```python
from build123d import *

# Parameters (mm, degrees)
ESBO_O1_R                  = 25
RESSALTO_EXTRUS_O1_DEPTH   = 30
ESBO_O2_R                  = 35
CORTE_EXTRUS_O1_DEPTH      = 25
ESBO_O3_R                  = 2.9
RESSALTO_EXTRUS_O2_DEPTH   = 6
ESBO_O4_R                  = 3
CORTE_EXTRUS_O2_DEPTH      = 123.727390525
CORTE_EXTRUS_O3_REACH      = 189.931
PADR_OCIRCULAR1_COUNT      = 9
CORTE_EXTRUS_O4_DEPTH      = 123.975657693
CORTE_EXTRUS_O4_DEPTH_BACK = 123.975657693
ESBO_O7_W                  = 10
ESBO_O7_H                  = 6
ESBO_O7_W_2                = 12
ESBO_O7_H_2                = 15
FILETE1_R                  = 1


with BuildPart() as part:
    # Esboço1 → Ressalto-extrusão1 (new body)
    with BuildSketch(Plane(origin=(0, 0, 0), x_dir=(1, 0, 0), z_dir=(0, 1, 0))):
        Polygon((-73.430577701, 42.395163802), (-83.502172006, -14.723685872), (-54.502172006, -64.953159292), (0, -84.790327605), (54.502172006, -64.953159292), (83.502172006, -14.723685872), (73.430577701, 42.395163802), (29, 79.676845164), (-29, 79.676845164), align=None)
        with Locations(Location((0, 0, 0), (0, 0, 270))):
            Circle(ESBO_O1_R, mode=Mode.SUBTRACT)
    extrude(amount=RESSALTO_EXTRUS_O1_DEPTH)

    # Esboço2 → Corte-extrusão1 (cut)
    with BuildSketch(Plane(origin=(0, 30, 0), x_dir=(1, 0, 0), z_dir=(0, 1, 0))):
        Polygon((-79.310129922, -13.984515749), (-51.766010859, -61.692329415), (0, -80.533616515), (51.766010859, -61.692329415), (79.310129922, -13.984515749), (69.74415776, 40.266808257), (27.544119063, 75.676845164), (-27.544119063, 75.676845164), (-69.74415776, 40.266808257), align=None)
        with Locations(Location((0, 0, 0), (0, 0, 270))):
            Circle(ESBO_O2_R, mode=Mode.SUBTRACT)
    extrude(amount=-CORTE_EXTRUS_O1_DEPTH, mode=Mode.SUBTRACT)

    # Esboço3 → Ressalto-extrusão2 (add)
    with BuildSketch(Plane(origin=(0, 30, 0), x_dir=(1, 0, 0), z_dir=(0, 1, 0))):
        with Locations(Location((0, 30, 0), (0, 0, 90))):
            Circle(ESBO_O3_R)
        with Locations(Location((25.980762114, -15, 0), (0, 0, 90))):
            Circle(ESBO_O3_R)
        with Locations(Location((-25.980762114, -15, 0), (0, 0, 90))):
            Circle(ESBO_O3_R)
    extrude(amount=RESSALTO_EXTRUS_O2_DEPTH)

    # Esboço4 → Corte-extrusão2 (cut, through all)
    with BuildSketch(Plane(origin=(0, 30, 0), x_dir=(1, 0, 0), z_dir=(0, 1, 0))):
        with Locations(Location((0, -30, 0), (0, 0, 270))):
            Circle(ESBO_O4_R)
        with Locations(Location((-25.980762114, 15, 0), (0, 0, 270))):
            Circle(ESBO_O4_R)
        with Locations(Location((25.980762114, 15, 0), (0, 0, 270))):
            Circle(ESBO_O4_R)
    extrude(amount=-CORTE_EXTRUS_O2_DEPTH, mode=Mode.SUBTRACT)

    # Esboço5 → Corte-extrusão3 (cut, up to next)
    with BuildSketch(Plane(origin=(0, 0, -79.676845164), x_dir=(-1, 0, 0), z_dir=(0, 0, -1)), mode=Mode.PRIVATE) as corte_extrus_o3_sk1:
        with BuildLine():
            Line((-14.5, 22.5), (14.5, 22.5))
            ThreePointArc((14.5, 22.5), (22, 15), (14.5, 7.5))
            Line((14.5, 7.5), (-14.5, 7.5))
            ThreePointArc((-14.5, 7.5), (-22, 15), (-14.5, 22.5))
        make_face()
    corte_extrus_o3_tool1 = extrude(corte_extrus_o3_sk1.sketch, amount=-CORTE_EXTRUS_O3_REACH, mode=Mode.PRIVATE) & part.part
    corte_extrus_o3 = corte_extrus_o3_tool1.solids().sort_by_distance((0, 15, -79.676845))[0]
    add(corte_extrus_o3, mode=Mode.SUBTRACT)

    # PadrãoCircular1: Corte-extrusão3 ×9 about axis
    padr_ocircular1_axis = Axis((0, 0, 0), (0, 1, 0))
    for i in range(1, PADR_OCIRCULAR1_COUNT):
        add(corte_extrus_o3.rotate(padr_ocircular1_axis, i * 360 / PADR_OCIRCULAR1_COUNT), mode=Mode.SUBTRACT)

    # Esboço7 → Corte-extrusão4 (cut, two sides: drawn at the far end of the back side and taken through both)
    with BuildSketch(Plane(origin=(0, 5, 0), x_dir=(1, 0, 0), z_dir=(0, 1, 0)).offset(-CORTE_EXTRUS_O4_DEPTH_BACK)):
        Polygon((30.672588783, 44.332787011), (38.333033214, 37.904910914), (42.189758872, 42.501177572), (34.529314441, 48.929053669), align=None)
        with Locations((0, 56.676845164)):
            Rectangle(ESBO_O7_W, ESBO_O7_H)
        Polygon((51.993132387, 14.244925111), (53.729614163, 4.396847581), (59.638460681, 5.438736647), (57.901978905, 15.286814177), align=None)
        Polygon((48.985511507, -22.508295563), (43.985511507, -31.168549601), (49.18166393, -34.168549601), (54.18166393, -25.508295563), align=None)
        Polygon((23.05702538, -48.729634591), (13.660099172, -52.149836024), (15.712220032, -57.787991749), (25.10914624, -54.367790316), align=None)
        Polygon((-13.660099172, -52.149836024), (-23.05702538, -48.729634591), (-25.10914624, -54.367790316), (-15.712220032, -57.787991749), align=None)
        Polygon((-43.985511507, -31.168549601), (-48.985511507, -22.508295563), (-54.18166393, -25.508295563), (-49.18166393, -34.168549601), align=None)
        Polygon((-53.729614163, 4.396847581), (-51.993132387, 14.244925111), (-57.901978905, 15.286814177), (-59.638460681, 5.438736647), align=None)
        Polygon((-38.333033214, 37.904910914), (-30.672588783, 44.332787011), (-34.529314441, 48.929053669), (-42.189758872, 42.501177572), align=None)
        Polygon((-23.065208837, -36.822388457), (-32.257742154, -29.10893714), (-41.8995563, -40.599603787), (-32.707022982, -48.313055103), align=None)
        with Locations((0, -50.533616515)):
            Rectangle(ESBO_O7_W_2, ESBO_O7_H_2)
        Polygon((-41.337950118, -13.381555604), (-43.42172825, -1.563862568), (-58.193844545, -4.168585233), (-56.110066413, -15.986278269), align=None)
        Polygon((-40.268205119, 16.320655835), (-34.268205119, 26.71296068), (-47.258586175, 34.21296068), (-53.258586175, 23.820655835), align=None)
        Polygon((-20.356519413, 38.386251025), (-9.080207964, 42.490492745), (-14.210510113, 56.585882056), (-25.486821563, 52.481640337), align=None)
        Polygon((9.080207964, 42.490492745), (20.356519413, 38.386251025), (25.486821563, 52.481640337), (14.210510113, 56.585882056), align=None)
        Polygon((34.268205119, 26.71296068), (40.268205119, 16.320655835), (53.258586175, 23.820655835), (47.258586175, 34.21296068), align=None)
        Polygon((43.42172825, -1.563862568), (41.337950118, -13.381555604), (56.110066413, -15.986278269), (58.193844545, -4.168585233), align=None)
        Polygon((32.257742154, -29.10893714), (23.065208837, -36.822388457), (32.707022982, -48.313055103), (41.8995563, -40.599603787), align=None)
    extrude(amount=CORTE_EXTRUS_O4_DEPTH + CORTE_EXTRUS_O4_DEPTH_BACK, mode=Mode.SUBTRACT)

    # Filete1
    filete1_edges = [part.edges().sort_by_distance(p)[0] for p in [
        (0, 36, -27.1),
        (25.980762114, 36, 17.9),
        (-25.980762114, 36, 17.9),
    ]]
    fillet(filete1_edges, radius=FILETE1_R)


solid = part.part
```
CAD build for the part. Positions are in the model's coordinates, mm. A direction names the side the tool comes from. Coordinates: 2 decimals unless noted, no trailing zeros. Return JSON: item names as keys, results as strings.
1. Mould opens along Y. For faces 6 (the flat face through (-26, 7.5, 73)), 7 (the flat face through (78.537, 24.79, -13.436)) say: released by +Y, released by -Y, zero draft, split by the parting line, or undercut.
Result:
{"face 6": "undercut", "face 7": "zero draft"}
2. Drop flat-ended pins along their axis: pin 1 (10 mm diameter, centred on x = -62.5, z = 43, fed in from +Y); pin 2 (10 mm diameter, centred on y = 8, z = -34, fed in from -X); pin 3 (1.5 mm diameter, centred on y = 2, z = -55.5, fed in from +X). Give the stop position or say it passes through.
Result:
{"pin 1": "stops at y = 30", "pin 2": "stops at x = -75.79", "pin 3": "stops at x = 58.71"}
3. 3-axis set-ups, long thin cutter, end or side, ignore diameter. For faces 1 (the cylindrical face through (80.34, 14.84, 8.17)), 2 (the flat face through (-78.396, 24.79, -14.236)), 3 (the flat face through (-56.725, 2.465, -4.925)), 4 (the flat face through (48.94, 23.231, -57.724)), 5 (the flat face through (77, 22.5, -13)): which of +Z, -Z, +X, -X, +Y, -Y reach the whole face in a straight line?
Result:
{"face 1": "-Z", "face 2": "-Z, -X, +Y, -Y", "face 3": "+Y, -Y", "face 4": "+Y", "face 5": "+X"}
4. Band-saw the part on A-A (y = 15). State how many separate pieces and enclosed holes the cut face has, and give its area (3 significant figures).
Result:
{"separate pieces": "10", "enclosed holes": "4", "area": "2,250 mm2"}
5. Probe L1, parallel to Y at x = 59.5, z = -52.5; L2, parallel to X at y = 23.5, z = 9.5; L3, parallel to X at y = 22, z = -15. List the from-to ranges inside material, lowest first. Write a range as from..to.
Result:
{"L1": "y = 0..7.5, 22.5..30", "L2": "x = -82.58..-78.52, -33.69..-23.12, 23.12..33.69, 78.52..82.58", "L3": "x = -31.62..-28.98, -22.98..-20, 20..22.98, 28.98..31.62"}
